Read the model definition and answer for the solid it produces. Units are mm, in the model's axes. Round coordinates to 2 decimals unless told otherwise and drop trailing zeros. Loops run counter-clockwise (first coordinate to the right, second up) from the corner with the lowest first, then second, coordinate; pieces in that order, holes last. Notation, with made-up numbers: M 55.25,-6.75 L 96.25,-6.75 A19 cw 96.25,-0.75 Z; hole C 13,-21 d11. An arc over 180 degrees is marked long. Write each question's results on one line, items separated by ' | '.
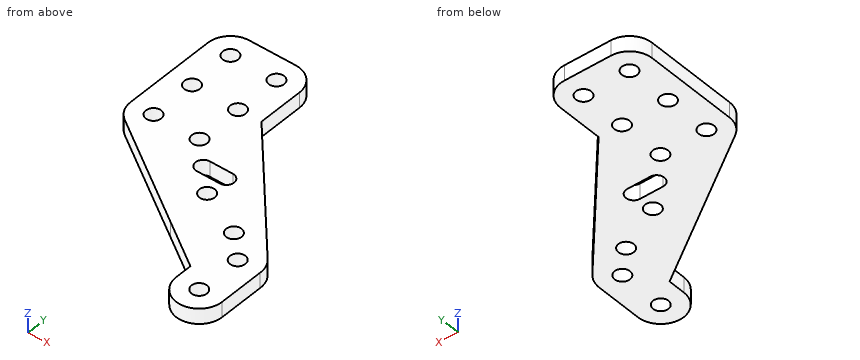
```python
from build123d import *

# Parameters (mm, degrees)
MODEL_R                 = 1.5
SALIENTE_EXTRUIR1_DEPTH = 3


with BuildPart() as part:
    # Model → Saliente-Extruir1 (new body)
    with BuildSketch(Plane.XY):
        with BuildLine():
            Line((47.956564936, 294.416156902), (47.956564936, 276.316156902))
            ThreePointArc((47.956564936, 276.316156902), (48.482384187, 274.205259611), (49.936959325, 272.587673623))
            Line((49.936959325, 272.587673623), (70.456564936, 258.72109315))
            Line((70.456564936, 258.72109315), (79.456564936, 252.639142716))
            Line((79.456564936, 252.639142716), (79.456564936, 249.316156902))
            ThreePointArc((79.456564936, 249.316156902), (83.956564936, 244.816156902), (88.456564936, 249.316156902))
            Line((88.456564936, 249.316156902), (88.456564456, 249.318235809))
            Line((88.456564456, 249.318235809), (88.454517382, 258.180422621))
            ThreePointArc((88.454517382, 258.180422621), (88.187667044, 259.848401972), (87.32462533, 261.300477459))
            Line((87.32462533, 261.300477459), (65.956564936, 285.416156902))
            Line((65.956564936, 285.416156902), (65.956564936, 294.316156902))
            ThreePointArc((65.956564936, 294.316156902), (64.638545451, 297.498137417), (61.456564936, 298.816156902))
            Line((61.456564936, 298.816156902), (52.356564936, 298.816156902))
            ThreePointArc((52.356564936, 298.816156902), (49.245295099, 297.527426739), (47.956564936, 294.416156902))
        make_face()
        with Locations((83.956564936, 249.316156902)):
            Circle(MODEL_R, mode=Mode.SUBTRACT)
        with Locations((70.456564936, 267.316156902)):
            Circle(MODEL_R, mode=Mode.SUBTRACT)
        with Locations((79.456564936, 262.816156902)):
            Circle(MODEL_R, mode=Mode.SUBTRACT)
        with Locations((83.956564936, 258.316156902)):
            Circle(MODEL_R, mode=Mode.SUBTRACT)
        with Locations((52.456564936, 276.316156902)):
            Circle(MODEL_R, mode=Mode.SUBTRACT)
        with Locations((61.456564936, 276.316156902)):
            Circle(MODEL_R, mode=Mode.SUBTRACT)
        with BuildLine():
            ThreePointArc((65.956564936, 270.316156902), (64.456564936, 271.816156902), (65.956564936, 273.316156902))
            Line((65.956564936, 273.316156902), (70.456564936, 273.316156902))
            ThreePointArc((70.456564936, 273.316156902), (71.956564936, 271.816156902), (70.456564936, 270.316156902))
            Line((70.456564936, 270.316156902), (65.956564936, 270.316156902))
        make_face(mode=Mode.SUBTRACT)
        with Locations((52.456564936, 285.316156902)):
            Circle(MODEL_R, mode=Mode.SUBTRACT)
        with Locations((52.456564936, 294.316156902)):
            Circle(MODEL_R, mode=Mode.SUBTRACT)
        with Locations((61.456564936, 285.316156902)):
            Circle(MODEL_R, mode=Mode.SUBTRACT)
        with Locations((61.456564936, 294.316156902)):
            Circle(MODEL_R, mode=Mode.SUBTRACT)
    extrude(amount=SALIENTE_EXTRUIR1_DEPTH)


solid = part.part
```
1. Find the intervals of material crossed by L1, parallel to X at y = 275.5, z = 1.05; L2, parallel to Y at x = 71, z = 1.7; L3, parallel to X at y = 294, z = 1.8, in increasing order.
Completed:
L1: x = 48.03 to 51.2, 53.72 to 60.2, 62.72 to 74.74 | L2: y = 258.35 to 265.92, 268.71 to 270.42, 273.21 to 279.72 | L3: x = 47.96 to 50.99, 53.92 to 59.99, 62.92 to 65.96
2. Find section A-A, the plane z = 1.9. Count the separate pieces of the cut face and the enclosed holes in it, then the cut area to 3 significant figures.
Completed:
separate pieces: 1 | enclosed holes: 11 | area: 908 mm2
3. Find section C-C, the plane y = 287.5. Give the vertices of the cut face in (x, z).
Completed:
outline: M 47.96,0 L 65.96,0 L 65.96,3 L 47.96,3 Z
4. Find section D-D, the plane x = 59. Give the vertices of the cut face in (y, z).
Completed:
outline: M 266.46,0 L 298.82,0 L 298.82,3 L 266.46,3 Z
5. Find section B-B, the plane x = 78.5. Give the vertices of the cut face in (y, z), then the cut area to 3 significant figures.
Completed:
outline: M 253.29,0 L 261.66,0 L 261.66,3 L 253.29,3 Z; M 263.97,0 L 271.26,0 L 271.26,3 L 263.97,3 Z | area: 47.0 mm2
6. Given P1, Ø1.5, axis at y = 262, z = 2.5, coming from the +X side; P2, Ø1.5, axis at y = 290.5, z = 2, coming from the +X side; P3, Ø1, axis at x = 70.5, z = 1.5, coming from the +Y side, each flat-ended and moving along its own axis, determine where each tip first touches the part or whether it passes through.
Completed:
P1: stops at x = 87.37 | P2: stops at x = 65.96 | P3: stops at y = 280.85
